Answer from the drawing. Dimensions are ordinates in mm from the lowest x, y and z of the part. Coordinates: 2 decimals unless noted, no trailing zeros. Write each loop counter-clockwise with the first axis right and the second up, starting at its lowest first coordinate (ties: lowest second). Pieces come first, ordered by that corner, then holes. Notation, with made-up numbers: M -27,-27.75 L 2,-27.75 A26 ccw 2,-3.75 Z; hole C 33.25,-4.75 d11. An arc over 180 degrees is marked long. Put each result on its own line as item: value. Start each with the question number.
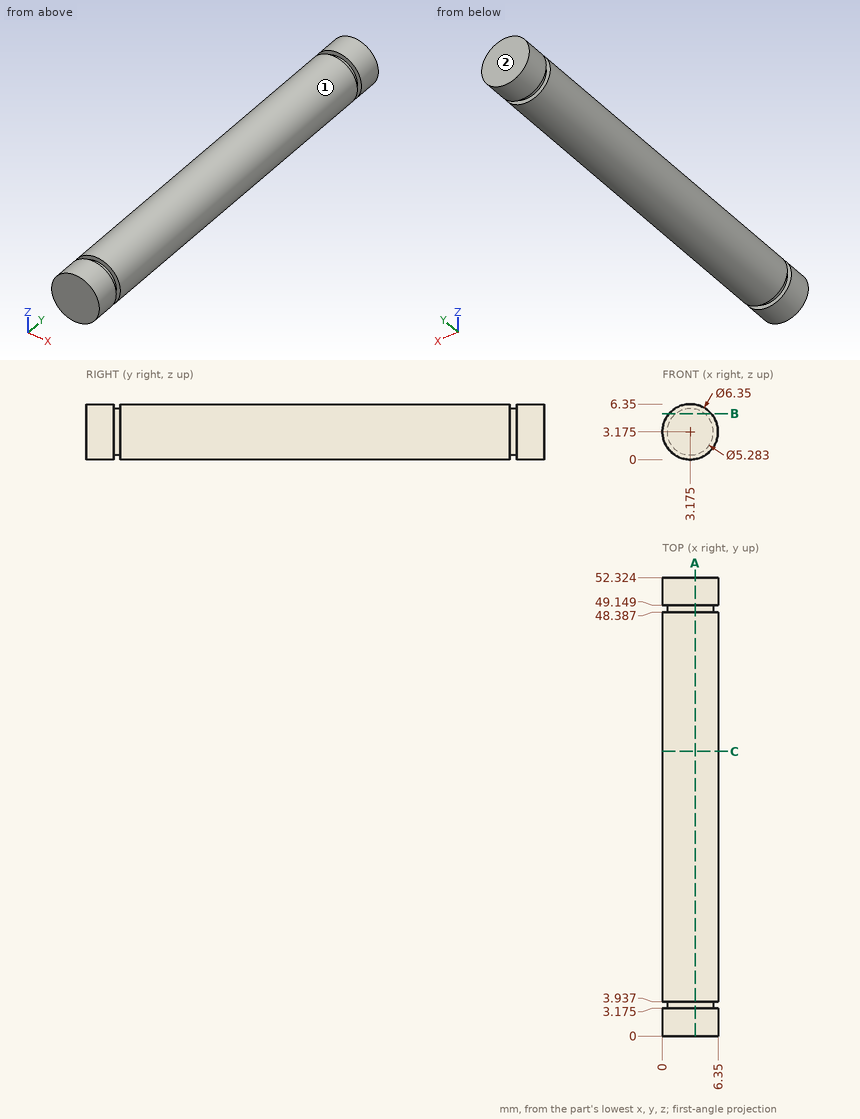
1) A cutting plane is placed at B-B on z = 5.25. Write down the section's boundary in (x, y) (1 decimal).
2) A cutting plane is placed at A-A on x = 3.75. Write down the section's boundary in (y, z) (1 decimal).
3) Straight lines are drawn through the part: probe 1 along Y at (x, z) = (5, 0.75) (3 decimals); probe 2 along X at (y, z) = (25, 3.25). For each, find the intervals that lie inside material, in ascending order.
4) A cutting plane is placed at C-C on y = 32.5. Write down the section's boundary in (x, z) (3 decimals), then the cut area to 3 significant figures.
5) Given pin 1 Ø2 at (x, y) = (4.5, 6.5) entering from -Z; pin 2 Ø3 at (y, z) = (45, 5) entering from -X, each flat-ended and moving along its own axis, determine where each tip first touches the part or whether it passes through.
6) Determine the mould class of the marked faces 1 and 2 for opening direction Z: +Z half, -Z half, draft (parallel to the pull), parting line (faces both ways), or undercut.
Answers follow:
1. outline: M 0.8,0 L 5.6,0 L 5.6,3.2 L 4.8,3.2 L 4.8,3.9 L 5.6,3.9 L 5.6,48.4 L 4.8,48.4 L 4.8,49.1 L 5.6,49.1 L 5.6,52.3 L 0.8,52.3 L 0.8,49.1 L 1.5,49.1 L 1.5,48.4 L 0.8,48.4 L 0.8,3.9 L 1.5,3.9 L 1.5,3.2 L 0.8,3.2 Z
2. outline: M 0,0.1 L 3.2,0.1 L 3.2,0.6 L 3.9,0.6 L 3.9,0.1 L 48.4,0.1 L 48.4,0.6 L 49.1,0.6 L 49.1,0.1 L 52.3,0.1 L 52.3,6.3 L 49.1,6.3 L 49.1,5.8 L 48.4,5.8 L 48.4,6.3 L 3.9,6.3 L 3.9,5.8 L 3.2,5.8 L 3.2,6.3 L 0,6.3 Z
3. probe 1: y = 0 to 3.175, 3.937 to 48.387, 49.149 to 52.324
3. probe 2: x = 0 to 6.35
4. outline: C 3.175,3.175 d6.35
4. area: 31.7 mm²
5. pin 1: stops at z = 0.02
5. pin 2: stops at x = 0.02
6. face 1: parting line
6. face 2: draft
